For this review, take the finished solid that the model builds, in its own axes (mm). Give positions to 0.01 mm unless a question says otherwise; leave off trailing zeros. Write each loop counter-clockwise with the first axis right and the second up, starting at its lowest first coordinate (ties: lowest second). Pieces come first, ordered by that corner, then holes. Notation, with made-up numbers: (84, 68.5) -> (103, 68.5) arc R23 ccw to (103, 94.5) -> close; hole circle Ø9 at (65, -36). An arc over 180 degrees is marked (long way). Return JSON: item names as keys, results as strings.
from build123d import *

# Parameters (mm, degrees)
SKETCH1_R                       = 266.7
BOSS_EXTRUDE1_DEPTH             = 5.842
SKETCH2_R                       = 2.5527
HOLES_MOUNTINGPOLARMECH_DEPTH   = 378.215997757
CUTOUT_STEPPERMOTORRELIEF_DEPTH = 378.215997757
FILLET_STEPPERMOTORRELIEF_R     = 5.08
SKETCH4_R                       = 2.5527
HOLES_FEET_DEPTH                = 378.215997757
CIRPATTERN_FEET_COUNT           = 5
SKETCH5_R                       = 2.5527
CUT_EXTRUDE1_DEPTH              = 378.215997757


with BuildPart() as part:
    # Sketch1 → Boss-Extrude1 (new body)
    with BuildSketch(Plane(origin=(0, 0, 0), x_dir=(1, 0, 0), z_dir=(0, 1, 0))):
        with Locations(Location((0, 0, 0), (0, 0, 270))):
            Circle(SKETCH1_R)
    extrude(amount=BOSS_EXTRUDE1_DEPTH)

    # Sketch2 → Holes-MountingPolarMech (cut, through all)
    with BuildSketch(Plane(origin=(0, 5.842, 0), x_dir=(1, 0, 0), z_dir=(0, 1, 0))):
        with Locations(Location((55.88, 54.61, 0), (0, 0, 270))):
            Circle(SKETCH2_R)
        with Locations(Location((-48.26, 64.77, 0), (0, 0, 270))):
            Circle(SKETCH2_R)
        with Locations(Location((-48.26, -64.77, 0), (0, 0, 270))):
            Circle(SKETCH2_R)
        with Locations(Location((55.88, -54.61, 0), (0, 0, 270))):
            Circle(SKETCH2_R)
        with Locations(Location((-123.19, 29.21, 0), (0, 0, 270))):
            Circle(SKETCH2_R)
        with Locations(Location((-123.19, -29.21, 0), (0, 0, 270))):
            Circle(SKETCH2_R)
    extrude(amount=-HOLES_MOUNTINGPOLARMECH_DEPTH, mode=Mode.SUBTRACT)

    # Sketch3 → Cutout-StepperMotorRelief (cut, through all)
    with BuildSketch(Plane(origin=(0, 5.842, 0), x_dir=(1, 0, 0), z_dir=(0, 1, 0))):
        Polygon((-123.19, 22.86), (-149.86, 22.86), (-149.86, 0), (-149.86, -22.86), (-123.19, -22.86), (-96.52, -22.86), (-96.52, -11.43), (-81.28, -11.43), (-81.28, 0), (-81.28, 11.43), (-96.52, 11.43), (-96.52, 22.86), align=None)
    extrude(amount=-CUTOUT_STEPPERMOTORRELIEF_DEPTH, mode=Mode.SUBTRACT)

    # Fillet-StepperMotorRelief
    fillet_steppermotorrelief_edges = [part.edges().sort_by_distance(p)[0] for p in [
        (-81.28, 2.921, -11.43),
        (-81.28, 2.921, 11.43),
        (-96.52, 2.921, 11.43),
        (-96.52, 2.921, 22.86),
        (-149.86, 2.921, 22.86),
        (-149.86, 2.921, -22.86),
        (-96.52, 2.921, -22.86),
        (-96.52, 2.921, -11.43),
    ]]
    fillet(fillet_steppermotorrelief_edges, radius=FILLET_STEPPERMOTORRELIEF_R)

    # Sketch4 → Holes-Feet (cut, through all)
    with BuildSketch(Plane(origin=(0, 5.842, 0), x_dir=(1, 0, 0), z_dir=(0, 1, 0))):
        with Locations(Location((250.19, 0, 0), (0, 0, 270))):
            Circle(SKETCH4_R)
        with Locations(Location((196.85, 0, 0), (0, 0, 270))):
            Circle(SKETCH4_R)
    holes_feet = extrude(amount=-HOLES_FEET_DEPTH, mode=Mode.SUBTRACT)

    # CirPattern-Feet: Holes-Feet ×5 about axis
    cirpattern_feet_axis = Axis((0, 0, 0), (0, 1, 0))
    for i in range(1, CIRPATTERN_FEET_COUNT):
        add(holes_feet.rotate(cirpattern_feet_axis, i * 360 / CIRPATTERN_FEET_COUNT), mode=Mode.SUBTRACT)

    # Sketch5 → Cut-Extrude1 (cut, through all)
    with BuildSketch(Plane.XZ):
        with Locations(Location((104.369393552, 218.470806035, 0), (0, 0, 270))):
            Circle(SKETCH5_R)
    extrude(amount=-CUT_EXTRUDE1_DEPTH, mode=Mode.SUBTRACT)


solid = part.part
1. For pin 1 (3 mm diameter, centred on y = 1, z = 90, fed in from -X); pin 2 (2.5 mm diameter, centred on x = -88.5, y = 2.5, fed in from -Z), all flat-tipped, find the tip position at first contact; note any pin that passes through.
Results found:
{"pin 1": "stops at x = -251.59", "pin 2": "stops at z = -252.02"}
2. To check wall thickness, follow probe 1 along X at (y, z) = (1.15, 4.5); probe 2 along X at (y, z) = (4.5, 54.61); probe 3 along Z at (x, y) = (-185.5, 0.7). State the ranges of each line that lie inside material, in increasing order.
Results found:
{"probe 1": "x = -266.66 to -149.86, -81.28 to 266.66", "probe 2": "x = -261.05 to 53.33, 58.43 to 261.05", "probe 3": "z = -191.62 to 191.62"}
3. Add section C-C, the plane x = 209.5. State the section outline as (y, z) points, plus the area to 3 significant figures.
Results found:
{"outline": "(0, -165.04) -> (5.84, -165.04) -> (5.84, 165.04) -> (0, 165.04) -> close", "area": "1,930 mm²"}
4. Add section B-B, the plane z = 94. State the section outline as (x, y) points, plus the area to 3 significant figures.
Results found:
{"outline": "(-249.59, 0) -> (249.59, 0) -> (249.59, 5.84) -> (-249.59, 5.84) -> close", "area": "2,920 mm²"}
5. Add section A-A, the plane y = 3.85. Count the separate pieces of the cut face and the enclosed holes in it, plus the area to 3 significant figures.
Results found:
{"separate pieces": "1", "enclosed holes": "18", "area": "220,000 mm²"}
